Autodesk Fusion 360 part; units mm, degrees
sketch "Sketch1" plane through (0, 0, 0) normal (0, 1, 0) x (1, 0, 0)
  line L0 (0, 0) -> (66, 0)
  line L1 (0, 0) -> (0, -8) construction
  line L2 (74, -8) -> (74, -73)
  line L3 (74, -73) -> (70, -73)
  line L4 (70, -73) -> (70, -79)
  line L5 (70, -79) -> (66, -79)
  line L6 (66, -79) -> (66, -16)
  line L7 (58, -8) -> (0, -8)
  arc A0 (66, -16) -> (58, -8) centre (58, -16) ccw
  arc A1 (74, -8) -> (66, 0) centre (66, -8) ccw
  line L8 (-58, -8) -> (0, -8)
  line L9 (0, 0) -> (-66, 0)
  arc A2 (-66, 0) -> (-74, -8) centre (-66, -8) ccw
  line L10 (-74, -8) -> (-74, -73)
  arc A3 (-58, -8) -> (-66, -16) centre (-58, -16) ccw
  line L11 (-66, -79) -> (-66, -16)
  line L12 (-70, -79) -> (-66, -79)
  line L13 (-70, -73) -> (-70, -79)
  line L14 (-74, -73) -> (-70, -73)
  circle A4 centre (0, -4) radius 1.5
  point P0 (74, 0)
  point P1 (66, -8)
  dimension "d1" = 74
  dimension "d2" = 8
  dimension "d3" = 73
  dimension "d4" = 4
  dimension "d5" = 6
  dimension "d6" = 4
  dimension "d7" = 71
  dimension "d8" = 8
  dimension "d9" = 8
  dimension "d10" = 3
extrude "Extrude1" add sketch "Sketch1" along normal blind 12
fillet "Fillet1" radius 6 4 edges at (68, 12, 79) (68, 0, 79) (-68, 12, 79) (-68, 0, 79)
sketch "Sketch2" plane through (-74, 0, 0) normal (1, 0, 0) x (0, 1, 0)
  arc A0 (12, 73) -> (0, 73) centre (6, 73) ccw
  line L0 (0, 73) -> (0, 16)
  line L1 (0, 16) -> (12, 16)
  line L2 (12, 16) -> (12, 73)
  line L3 (6, 16) -> (6, 71) construction
  circle A1 centre (6, 71) radius 4.5
  line L4 (0, 8) -> (0, 73)
  line L5 (0, 73) -> (12, 73)
  line L6 (12, 73) -> (12, 8)
  line L7 (12, 8) -> (0, 8)
  dimension "d15" = 55
  dimension "d16" = 9
hole "Hole1" at (-74, 6, 71) direction (1, 0, 0) diameter 9 depth 10 tip angle 118 counterbore diameter 10 counterbore depth 4
mirror "Mirror1" about plane through (0, 0, 0) normal (1, 0, 0) of "Hole1"
sketch "Sketch3" plane through (0, 0, 8) normal (0, 0, 1) x (-1, 0, 0)
  line L0 (58, 0) -> (-58, 0)
  line L1 (-58, 0) -> (-58, -12)
  line L2 (-58, -12) -> (58, -12)
  line L3 (58, -12) -> (58, 0)
  line L4 (0, 0) -> (0, -6) construction
  circle A0 centre (0, -6) radius 3
  dimension "d24" = 6
  dimension "d25" = 6
hole "Hole2" at (0, 6, 8) direction (0, 0, -1) diameter 6 depth 10 tip angle 118
Work out the finished part from the listing and answer in its coordinate system (mm). A direction names the side the tool comes from. Give positions to 0.01 mm unless a question says otherwise; leave off trailing zeros. Loops run counter-clockwise (first coordinate to the right, second up) from the corner with the lowest first, then second, coordinate; pieces in that order, holes last. Notation, with made-up numbers: (3, 36.5) - (52, 36.5) arc R17 cw to (52, 65.5) - close; hole circle Ø7 at (61.25, -4). An arc over 180 degrees is marked (long way). Answer in a Markdown table with one row per item. Add a question column.
Q1. A tool of negligible diameter and unlimited length cuts with its end or side. For faces 1 (the cylindrical face through (-67.972, 1.804, 77.289)), 2 (the cylindrical face through (63.594, 5.916, 10.281)), from which of +Z, -Z, +X, -X, +Y, -Y can it reach the whole face along a straight path? Write none if from no direction.
Q2. The part is cut by section C-C (z = 38.5). Determine the outline of the cut face in (x, y), and give its area (3 significant figures).
Q3. Determine the mould class of faces 3 (the cylindrical face through (-72, 6, 66)), 4 (the cylindrical face through (67.972, 10.196, 77.289)), 5 (the flat face through (-66, 6, 48)) for opening direction Z: released by +Z, released by -Z, zero draft, split by the parting line, or undercut.
Q4. Consider line 1 along X through (y, z) = (4.5, 24.5); line 2 along Y through (x, z) = (73, 71); line 3 along Y through (x, z) = (0, 6). Determine where each line is inside the solid, lowest interval first.
Q5. Each of these flat-tipped pins is pushed along its axis until it touches: P1, Ø3.5, axis at x = 20.5, y = 3, coming from the +Z side; P2, Ø1.1, axis at x = 71.5, y = 0.5, coming from the +Z side. Where does it stop, or does it pass through?
Q6. The part is cut by section D-D (z = 11.5). Determine the outline of the cut face in (x, y).
Q7. The part is cut by section B-B (x = 0). Determine the outline of the cut face in (y, z).
Q8. The part is cut by section A-A (z = 71). Determine the outline of the cut face in (x, y), and give its area (3 significant figures).
Solution:
| question | item | result |
|---|---|---|
| 1 | face 1 | +Z, +X, -X, -Y |
| 1 | face 2 | +Z, +Y, -Y |
| 2 | outline | (-74, 0) - (-66, 0) - (-66, 12) - (-74, 12) - close; (66, 0) - (74, 0) - (74, 12) - (66, 12) - close |
| 2 | area | 192 mm² |
| 3 | face 3 | undercut |
| 3 | face 4 | released by +Z |
| 3 | face 5 | zero draft |
| 4 | line 1 | x = -74 to -66, 66 to 74 |
| 4 | line 2 | y = 0 to 1, 11 to 12 |
| 4 | line 3 | y = 0 to 3, 9 to 12 |
| 5 | P1 | stops at z = 8 |
| 5 | P2 | stops at z = 73 |
| 6 | outline | (-74, 0) - (-64.61, 0) - (-64.61, 12) - (-74, 12) - close; (64.61, 0) - (74, 0) - (74, 12) - (64.61, 12) - close |
| 7 | outline | (0, 0) - (3, 0) - (3, 2.5) - (0, 2.5) - close; (0, 5.5) - (3, 5.5) - (3, 8) - (0, 8) - close; (9, 0) - (12, 0) - (12, 2.5) - (9, 2.5) - close; (9, 5.5) - (12, 5.5) - (12, 8) - (9, 8) - close |
| 8 | outline | (-74, 0) - (-66, 0) - (-66, 1.5) - (-70, 1.5) - (-70, 1) - (-74, 1) - close; (-74, 11) - (-70, 11) - (-70, 10.5) - (-66, 10.5) - (-66, 12) - (-74, 12) - close; (66, 0) - (74, 0) - (74, 1) - (70, 1) - (70, 1.5) - (66, 1.5) - close; (66, 10.5) - (70, 10.5) - (70, 11) - (74, 11) - (74, 12) - (66, 12) - close |
| 8 | area | 40.0 mm² |
